Part model, mm, in its own coordinate system. A direction names the side the tool comes from. Round coordinates to 2 decimals unless told otherwise and drop trailing zeros. Write each loop counter-clockwise with the first axis right and the second up, starting at its lowest first coordinate (ties: lowest second). Pieces come first, ordered by that corner, then holes.
1) Saw through at C-C on z = 8. Write the cut outline in (x, y), and give its area (3 significant figures).
2) Flat gauge pins, fed straight in: pin 1 (1.5 mm diameter, centred on x = -3.5, y = 22.5, fed in from -Z); pin 2 (2.5 mm diameter, centred on x = -3.5, y = 2, fed in from -Z); pin 3 (5 mm diameter, centred on y = 25, z = -8.5, fed in from +X); pin 4 (1.5 mm diameter, centred on x = -11, z = -5, fed in from -Y). Where does each tip first touch, or does it go through?
3) Drill centre lines: L1, parallel to Y at x = -11.5, z = 7; L2, parallel to Z at x = -4.5, y = 24; L3, parallel to Z at x = -13.5, y = 54.5. Where is each one in solid material? Low to high.
4) Saw through at A-A on x = -15. Write the cut outline in (y, z), and give its area (3 significant figures).
5) Saw through at D-D on x = -4. Write the cut outline in (y, z), and give its area (3 significant figures).
6) Saw through at B-B on y = 22. Write the cut outline in (x, z), and give its area (3 significant figures).
7) Pull direction X, two halves, no side cores. Call faces 4 (the flat face through (-3.843, 2.465, -2.344)), 5 (the flat face through (-10.977, 34.51, -5.988)), 6 (the flat face through (0, 70, -2)), 7 (the flat face through (0, 2, 4.5)): +X half, -X half, draft (parallel to the pull), parting line (faces both ways), or undercut.
8) Which spindle directions (+Z, -Z, +X, -X, +Y, -Y) get a long thin tool onto all of the face, cutting with end or side? Do faces 1 (the flat face through (10.674, 34.51, -6.512)), 2 (the flat face through (3.95, 2.46, -2.16)), 3 (the flat face through (0, 35, 9.5)). Say none if no direction does.
```python
from build123d import *

# Parameters (mm, degrees)
EXTRUDE_1_DEPTH = 70
EXTRUDE_2_DEPTH = 5
EXTRUDE_3_DEPTH = 5


with BuildPart() as part:
    # 草图1 → 凸台-拉伸1 (new body)
    with BuildSketch(Plane(origin=(0, 0, 0), x_dir=(1, 0, 0), z_dir=(0, 1, 0))):
        Polygon((0, 25), (21.650635095, -12.5), (-21.650635095, -12.5), align=None)
        Polygon((-16.454482672, -9.5), (0, 19), (16.454482672, -9.5), align=None, mode=Mode.SUBTRACT)
    extrude(amount=EXTRUDE_1_DEPTH)

    # 草图2 → 凸台-拉伸2 (add)
    with BuildSketch(Plane(origin=(0, 70, 0), x_dir=(1, 0, 0), z_dir=(0, 1, 0))):
        Polygon((0, 19), (16.454482672, -9.5), (-16.454482672, -9.5), align=None)
    extrude(amount=-EXTRUDE_2_DEPTH)

    # 草图3 → 凸台-拉伸3 (add)
    with BuildSketch(Plane.XZ):
        Polygon((-16.454482672, 9.5), (16.454482672, 9.5), (0, -19), align=None)
        Polygon((0, -9), (-7.794228634, 4.5), (7.794228634, 4.5), align=None, mode=Mode.SUBTRACT)
    extrude(amount=-EXTRUDE_3_DEPTH)


solid = part.part
```
Completed:
1. outline: (-19.05, 0) - (19.05, 0) - (19.05, 70) - (-19.05, 70) - close; hole (-15.59, 5) - (15.59, 5) - (15.59, 65) - (-15.59, 65) - close
1. area: 797 mm2
2. pin 1: stops at z = -20.24
2. pin 2: stops at z = -21.1
2. pin 3: stops at x = 10.97
2. pin 4: stops at y = 0
3. L1: y = 0 to 5, 65 to 70
3. L2: z = -17.21 to -11.21, 9.5 to 12.5
3. L3: z = -1.62 to 4.38, 9.5 to 12.5
4. outline: (0, 0.98) - (70, 0.98) - (70, 12.5) - (0, 12.5) - close; hole (5, 6.98) - (65, 6.98) - (65, 9.5) - (5, 9.5) - close
4. area: 655 mm2
5. outline: (0, -18.07) - (70, -18.07) - (70, 12.5) - (0, 12.5) - (0, 4.5) - (5, 4.5) - (5, 9.5) - (65, 9.5) - (65, -12.07) - (5, -12.07) - (5, -2.07) - (0, -2.07) - close
5. area: 813 mm2
6. outline: (-21.65, 12.5) - (0, -25) - (21.65, 12.5) - close; hole (-16.45, 9.5) - (0, -19) - (16.45, 9.5) - close
6. area: 343 mm2
7. face 4: undercut
7. face 5: -X half
7. face 6: draft
7. face 7: undercut
8. face 1: -Z, +X, +Y, -Y
8. face 2: -Y
8. face 3: none
